Autodesk Inventor part; units mm, degrees
ref_plane "YZ Plane" through (0, 0, 0) normal (1, 0, 0) x (0, 1, 0)
ref_plane "XZ Plane" through (0, 0, 0) normal (0, 1, 0) x (-1, 0, 0)
ref_plane "XY Plane" through (0, 0, 0) normal (0, 0, 1) x (1, 0, 0)
sketch "Sketch1" plane through (0, 0, 0) normal (1, 0, 0) x (0, 1, 0)
  arc A0 (37.5, 0) -> (15.0255, 34.3582) centre (0, 0) ccw
  circle A1 centre (15.0255, 34.3582) radius 4
  circle A2 centre (37.5, 0) radius 4
  arc A3 (33.5, 0) -> (13.4227, 30.6933) centre (0, 0) ccw
  arc A4 (41.5, 0) -> (16.6282, 38.0231) centre (0, 0) ccw
  arc A5 (30.9, 0) -> (44.1, 0) centre (37.5, 0) ccw
  arc A6 (17.6699, 40.4052) -> (12.381, 28.3112) centre (15.0255, 34.3582) ccw
  arc A7 (30.9, 0) -> (12.381, 28.3112) centre (0, 0) ccw
  arc A8 (44.1, 0) -> (17.6699, 40.4052) centre (0, 0) ccw
  circle A9 centre (37.5, 0) radius 1.25
  circle A10 centre (15.051, 34.347) radius 1.25
  arc A11 (36.0575, 3.7308) -> (17.8657, 31.5417) centre (0, 0) ccw
  arc A12 (38.5575, 3.8577) -> (18.9837, 33.7814) centre (0, 0) ccw
  dimension "d2" = 8
  dimension "d3" = 8
  dimension "d4" = 83
  dimension "d7" = 13.2
  dimension "d8" = 13.2
  dimension "d9" = 88.2
  dimension "d15" = 2.5
  dimension "d16" = 2.5
  dimension "d17" = 77.5
extrude "Extrusion1" add sketch "Sketch1" along normal blind 100.5 contours A2 A11 A1 A0 | A0 A1 A12 A2 | A2 | A1 | A9 | A10
extrude "Extrusion2" add sketch "Sketch1" against normal blind 3 contours A2 A11 A1 A0 | A0 A1 A12 A2 | A2 | A1 | A12 A1 A4 A2 | A2 A3 A1 A11 | A7 A6 A8 A5 | A9 | A10
fillet "Fillet1" radius 2 4 edges at (50.25, 36.0575, 3.7308) (50.25, 17.8657, 31.5417) (50.25, 18.9837, 33.7814) (50.25, 38.5575, 3.8577)
chamfer "Chamfer2" distance 0.8 angle 45 8 edges at (0, 37.7692, -3.9909) (0, 38.7564, 4.1228) (0, 32.4284, 21.2122) (0, 19.3063, 33.8574) (0, 11.4768, 36.204) (0, 18.0284, 31.1429) (0, 30.3363, 19.8437) (0, 35.7573, 4.0397)
sketch "Sketch2" plane through (100.5, 0, 0) normal (1, 0, 0) x (0, 0, -1)
  arc A0 (-34.7347, 19.0077) -> (-30.8815, 17.0036) centre (-34.3582, 15.0255) ccw
  arc A1 (-3.2054, 35.1072) -> (-3.4977, 39.4406) centre (0, 37.5) ccw
  circle A2 centre (-34.3582, 15.0255) radius 3.75
  circle A3 centre (0, 37.5) radius 3.75
  point P0 (0, 0)
  dimension "d22" = 7.5
  dimension "d23" = 7.5
extrude "Extrusion3" [suppressed]
sketch "Sketch3" plane through (102.8, 15.0255, 34.3582) normal (1, 0, 0) x (0, 0, -1)
  circle A0 centre (0, 0) radius 3.75
  circle A1 centre (0, 0) radius 4
  circle A2 centre (34.3582, 22.4745) radius 3.75
  circle A3 centre (34.3582, 22.4745) radius 4
  point P0 (34.3582, -15.0255)
  dimension "d26" = 8
  dimension "d27" = 8
extrude "Extrusion4" [suppressed]
chamfer "Chamfer3" [suppressed]
sketch "Sketch4" plane through (104.8, 15.0255, 34.3582) normal (1, 0, 0) x (0, 0, -1)
  circle A0 centre (34.3582, 22.4745) radius 2.5
  circle A1 centre (0, 0) radius 2.5
  arc A2 (34.3582, 22.4745) -> (0, 0) centre (34.3582, -15.0255) ccw
  line L0 (8.4634, -2.6098) -> (-7.662, 4.4422)
  line L1 (-7.662, 4.4422) -> (-8.4634, 2.6098)
  line L2 (-8.4634, 2.6098) -> (7.662, -4.4422)
  line L3 (7.662, -4.4422) -> (8.4634, -2.6098)
  line L4 (8.4634, -2.6098) -> (-8.4634, 2.6098) construction
  line L5 (-7.662, 4.4422) -> (7.662, -4.4422) construction
  line L6 (33.3582, 13.6745) -> (33.3582, 31.2745)
  line L7 (33.3582, 31.2745) -> (35.3582, 31.2745)
  line L8 (35.3582, 31.2745) -> (35.3582, 13.6745)
  line L9 (35.3582, 13.6745) -> (33.3582, 13.6745)
  line L10 (33.3582, 13.6745) -> (35.3582, 31.2745) construction
  line L11 (33.3582, 31.2745) -> (35.3582, 13.6745) construction
  point P0 (34.3582, -15.0255)
  point P1 (0, 0)
  dimension "d33" = 37.5
  dimension "d34" = 2
  dimension "d35" = 2
extrude "Extrusion5" [suppressed]
sketch "Sketch5" plane through (100.5, 0, 0) normal (1, 0, 0) x (0, 0, -1)
  arc A0 (-34.7347, 19.0077) -> (-30.8815, 17.0036) centre (-34.3582, 15.0255) ccw
  arc A1 (-3.2054, 35.1072) -> (-3.4977, 39.4406) centre (0, 37.5) ccw
  circle A2 centre (-34.3582, 15.0255) radius 2.85
  circle A3 centre (0, 37.5) radius 2.85
  point P0 (0, 0)
  dimension "d38" = 5.7
  dimension "d39" = 5.7
extrude "Extrusion6" cut sketch "Sketch5" against normal blind 4
sketch "Sketch6" plane through (96.5, 15.0255, 34.3582) normal (1, 0, 0) x (0, 0, -1)
  circle A0 centre (0, 0) radius 2.85
  circle A1 centre (34.3582, 22.4745) radius 2.85
  circle A2 centre (0, 0) radius 2.15
  circle A3 centre (34.3582, 22.4745) radius 2.15
  point P0 (34.3582, -15.0255)
  dimension "d42" = 4.3
  dimension "d43" = 4.3
extrude "Extrusion7" cut sketch "Sketch6" against normal blind 2 contours A2 | A3
equation "\"d23\" = d22"
equation "\"d35\" = d34"
properties part number "Mechanische_Anschlaege"
Can you work these out from the model? Positions are in its coordinate system, mm. A direction names the side the tool comes from. Give positions to 0.01 mm unless a question says otherwise; leave off trailing zeros. One line per item, written item: value.
1) We'd pull the mould along Z, two halves only. Please class faces 1 (the face through (98.53, 34.72, 0.62)), 2 (the face through (100.5, 31, 20)), 3 (the face through (-1.5, 26, 16.7)): released by +Z, released by -Z, zero draft, split by the parting line, or undercut.
Answer sheet:
face 1: undercut
face 2: zero draft
face 3: released by -Z
2) For P1, Ø5, axis at x = 53.5, y = 19, coming from the +Z side; P2, Ø5, axis at x = 42.5, y = 36, coming from the -Z side; P3, Ø1.7, axis at y = 37.5, z = -1, coming from the +X side, each with a flat end and sliding along its axis, tell me the tip position at first contact or that it passes through.
Answer sheet:
P1: stops at z = 38.08
P2: stops at z = -4
P3: stops at x = 94.5
3) Please list where these lines run through material, in increasing order: line 1 along Y through (x, z) = (7, 34.5); line 2 along X through (y, z) = (23.5, 21); line 3 along Z through (x, y) = (92, 15).
Answer sheet:
line 1: y = 11.03 to 19.04
line 2: x = -3 to 0
line 3: z = 30.36 to 38.36
4) On a 3-axis mill with a long thin cutter (end or side, diameter ignored), from which of +Z, -Z, +X, -X, +Y, -Y can I reach the whole of each face in a straight line? I mean faces 4 (the face through (95.51, 39.63, 0.28)), 5 (the face through (-3, 30, 18)). Say none if no direction works.
Answer sheet:
face 4: +X
face 5: +Z, -Z, -X, +Y, -Y
